Input: part model. Units: mm. Frame: model coordinates. A direction names the side the tool comes from. Coordinates: 2 decimals unless noted, no trailing zeros. Write each loop counter-clockwise with the first axis right and the second up, starting at its lowest first coordinate (ties: lowest second). Pieces come first, ordered by that corner, then holes. Notation, with made-up numbers: (7, 38) - (29, 38) arc R7 ccw to (29, 43) - close; hole circle Ø8 at (27.5, -13.75). An arc over 180 degrees is marked (long way). Use a Markdown table: item, result. Add a question column.
Q1. Section query A-A (y = 0). Return the cut outline in (x, z).
Q2. Mould query, pull axis X, two halves, no side actions, for faces 3 (the face through (0, 17.5, 1)), 4 (the face through (24.5, -8.5, 1.5)), 5 (the face through (31, 0, 1)). Classes: released by +X, released by -X, zero draft, split by the parting line, or undercut.
Q3. Material intervals for probe 1 along X at (y, z) = (-13.5, 1.95); probe 2 along Y at (x, z) = (27, 2.4); probe 3 along X at (y, z) = (0.5, 1.2), sorted ascending. Write a range as from..to.
Q4. Section query C-C (y = -12). Return the cut outline in (x, z).
Q5. Pin query (flat end, axial travel): P1, Ø2.5, axis at x = 27, y = 0, coming from the -Z side; P2, Ø1.3, axis at x = 24.5, z = 1.5, coming from the -Y side (3 decimals). Return the tip coordinate at first contact, or that it passes through.
Q6. Section query B-B (z = 0.45). Return the cut outline in (x, y).
Q7. Set-up query: faces 1 (the face through (0, -17.5, 1)), 2 (the face through (-26.15, -13, 1)). Return all of +Z, -Z, +X, -X, +Y, -Y with unobstructed straight access to the full face (end or side cutting, diameter ignored); none if empty.
from build123d import *

# Parameters (mm, degrees)
SKETCH_1_R      = 1.5
EXTRUDE_1_DEPTH = 3
FILLET_1_R      = 1


with BuildPart() as part:
    # 草图1 → 凸台-拉伸1 (new body)
    with BuildSketch(Plane.XY):
        Polygon((-31, -17.5), (-26.15, -17.5), (-26.15, -8.5), (-22.95, -8.5), (-22.95, -17.5), (22.95, -17.5), (22.95, -8.5), (26.15, -8.5), (26.15, -17.5), (31, -17.5), (31, 17.5), (-31, 17.5), align=None)
        with Locations((-27, 0)):
            Circle(SKETCH_1_R, mode=Mode.SUBTRACT)
        with Locations((27, 0)):
            Circle(SKETCH_1_R, mode=Mode.SUBTRACT)
    extrude(amount=EXTRUDE_1_DEPTH)

    # 圆角1
    fillet_1_edges = [part.edges().sort_by_distance(p)[0] for p in [
        (31, -17.5, 1.5),
        (26.15, -17.5, 1.5),
        (26.15, -8.5, 1.5),
        (22.95, -8.5, 1.5),
        (22.95, -17.5, 1.5),
        (-22.95, -17.5, 1.5),
        (-22.95, -8.5, 1.5),
        (-26.15, -8.5, 1.5),
        (-26.15, -17.5, 1.5),
        (-31, -17.5, 1.5),
        (-31, 17.5, 1.5),
        (31, 17.5, 1.5),
    ]]
    fillet(fillet_1_edges, radius=FILLET_1_R)


solid = part.part
Values follow:
| question | item | result |
|---|---|---|
| 1 | outline | (-31, 0) - (-28.5, 0) - (-28.5, 3) - (-31, 3) - close; (-25.5, 0) - (25.5, 0) - (25.5, 3) - (-25.5, 3) - close; (28.5, 0) - (31, 0) - (31, 3) - (28.5, 3) - close |
| 2 | face 3 | zero draft |
| 2 | face 4 | undercut |
| 2 | face 5 | released by +X |
| 3 | probe 1 | -31..-26.15, -22.95..22.95, 26.15..31 |
| 3 | probe 2 | -17.49..-1.5, 1.5..17.5 |
| 3 | probe 3 | -31..-28.41, -25.59..25.59, 28.41..31 |
| 4 | outline | (-31, 0) - (-26.15, 0) - (-26.15, 3) - (-31, 3) - close; (-22.95, 0) - (22.95, 0) - (22.95, 3) - (-22.95, 3) - close; (26.15, 0) - (31, 0) - (31, 3) - (26.15, 3) - close |
| 5 | P1 | through |
| 5 | P2 | y = -8.505 |
| 6 | outline | (-31, -16.5) arc R1 ccw to (-30, -17.5) - (-27.15, -17.5) arc R1 ccw to (-26.15, -16.5) - (-26.15, -9.5) arc R1 cw to (-25.15, -8.5) - (-23.95, -8.5) arc R1 cw to (-22.95, -9.5) - (-22.95, -16.5) arc R1 ccw to (-21.95, -17.5) - (21.95, -17.5) arc R1 ccw to (22.95, -16.5) - (22.95, -9.5) arc R1 cw to (23.95, -8.5) - (25.15, -8.5) arc R1 cw to (26.15, -9.5) - (26.15, -16.5) arc R1 ccw to (27.15, -17.5) - (30, -17.5) arc R1 ccw to (31, -16.5) - (31, 16.5) arc R1 ccw to (30, 17.5) - (-30, 17.5) arc R1 ccw to (-31, 16.5) - close; hole circle Ø3 at (-27, 0); hole circle Ø3 at (27, 0) |
| 7 | face 1 | +Z, -Z, +X, -X, -Y |
| 7 | face 2 | +Z, -Z, -Y |
